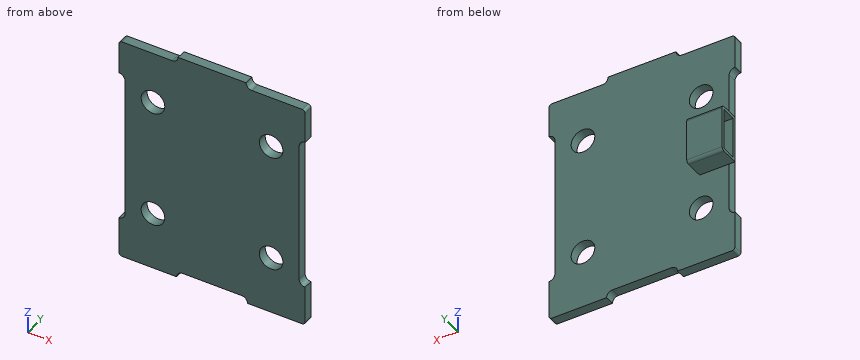
from build123d import *

# Parameters (mm, degrees)
SKETCH1_R           = 2
BOSS_EXTRUDE1_DEPTH = 1.6
SKETCH2_W           = 6
SKETCH2_H           = 8
BOSS_EXTRUDE2_DEPTH = 3.5
FILLET1_R           = 1
FILLET2_R           = 0.5
SKETCH3_W           = 7
SKETCH3_H           = 2.5
CUT_EXTRUDE1_DEPTH  = 5


with BuildPart() as part:
    # Sketch1 → Boss-Extrude1 (new body)
    with BuildSketch(Plane(origin=(0, 0, 0), x_dir=(1, 0, 0), z_dir=(0, 1, 0))):
        Polygon((15.75, 13), (15.75, 19.75), (6, 19.75), (6, 18.75), (-6, 18.75), (-6, 19.75), (-15.75, 19.75), (-15.75, 13), (-14.75, 13), (-14.75, -13), (-15.75, -13), (-15.75, -18.75), (-5.75, -18.75), (-5.75, -19.75), (5.75, -19.75), (5.75, -18.75), (15.75, -18.75), (15.75, -13), (14.75, -13), (14.75, 13), align=None)
        with Locations(Location((10, -10, 0), (0, 0, 270))):
            Circle(SKETCH1_R, mode=Mode.SUBTRACT)
        with Locations(Location((10, 10, 0), (0, 0, 270))):
            Circle(SKETCH1_R, mode=Mode.SUBTRACT)
        with Locations(Location((-10, 10, 0), (0, 0, 270))):
            Circle(SKETCH1_R, mode=Mode.SUBTRACT)
        with Locations(Location((-10, -10, 0), (0, 0, 270))):
            Circle(SKETCH1_R, mode=Mode.SUBTRACT)
    extrude(amount=BOSS_EXTRUDE1_DEPTH)

    # Sketch2 → Boss-Extrude2 (add)
    with BuildSketch(Plane(origin=(0, 1.6, 0), x_dir=(1, 0, 0), z_dir=(0, 1, 0))):
        with Locations((-12.75, 0)):
            Rectangle(SKETCH2_W, SKETCH2_H)
    extrude(amount=BOSS_EXTRUDE2_DEPTH)

    # Fillet1
    fillet1_edges = [part.edges().sort_by_distance(p)[0] for p in [
        (14.75, 0.8, -13),
        (14.75, 0.8, 13),
        (-6, 0.8, -18.75),
        (6, 0.8, -18.75),
        (-14.75, 0.8, -13),
        (-14.75, 0.8, 13),
        (-5.75, 0.8, 18.75),
        (5.75, 0.8, 18.75),
    ]]
    fillet(fillet1_edges, radius=FILLET1_R - 0.0001)  # a hair under: the kernel refuses the full size

    # Fillet2
    fillet2_edges = [part.edges().sort_by_distance(p)[0] for p in [
        (-15.75, 0.8, 18.75),
        (-15.75, 0.8, -19.75),
        (15.75, 0.8, -19.75),
        (15.75, 0.8, 18.75),
        (-12.75, 5.1, -4),
        (-12.75, 5.1, 4),
    ]]
    fillet(fillet2_edges, radius=FILLET2_R)

    # Sketch3 → Cut-Extrude1 (cut)
    with BuildSketch(Plane.ZY.offset(15.75)):
        with Locations((0, 3.35)):
            Rectangle(SKETCH3_W, SKETCH3_H)
    extrude(amount=-CUT_EXTRUDE1_DEPTH, mode=Mode.SUBTRACT)


solid = part.part
CAD build for the part. Positions are in the model's coordinates, mm. Give positions to 0.01 mm unless a question says otherwise; leave off trailing zeros. Order: outer loops, then holes, each group sorted by start corner. A loop starts at its lowest first (then second) coordinate and runs counter-clockwise, first axis right, second up. Notation, with made-up numbers: (41.5, 28.5) - (89.5, 28.5) arc R26 ccw to (89.5, 49.5) - close; hole circle Ø11 at (-0.5, 59.5). An arc over 180 degrees is marked (long way). Write each question's results on one line, items separated by ' | '.
1. Saw through at A-A on z = 10. List the corners of the cut face in (x, y), and give its area (3 significant figures).
Calculated:
outline: (-14.75, 0) - (-12, 0) - (-12, 1.6) - (-14.75, 1.6) - close; (-8, 0) - (8, 0) - (8, 1.6) - (-8, 1.6) - close; (12, 0) - (14.75, 0) - (14.75, 1.6) - (12, 1.6) - close | area: 34.4 mm2
2. Saw through at C-C on y = 3.65. List the corners of the cut face in (x, z).
Calculated:
outline: (-15.75, -4) - (-9.75, -4) - (-9.75, 4) - (-15.75, 4) - (-15.75, 3.5) - (-10.75, 3.5) - (-10.75, -3.5) - (-15.75, -3.5) - close
3. Saw through at D-D on z = -3. List the corners of the cut face in (x, y), and give its area (3 significant figures).
Calculated:
outline: (-15.75, 1.6) - (-14.75, 1.6) - (-14.75, 0) - (14.75, 0) - (14.75, 1.6) - (-9.75, 1.6) - (-9.75, 5.1) - (-15.75, 5.1) - (-15.75, 4.6) - (-10.75, 4.6) - (-10.75, 2.1) - (-15.75, 2.1) - close | area: 55.7 mm2
4. Probe L1, parallel to X at y = 0.9, z = -10; L2, parallel to Z at x = -11.5, y = 3.65; L3, parallel to X at y = 1.3, z = 9. List the from-to ranges inside material, lowest first. Write a range as from..to.
Calculated:
L1: x = -14.75..-12, -8..8, 12..14.75 | L2: z = -4..-3.5, 3.5..4 | L3: x = -14.75..-11.73, -8.27..8.27, 11.73..14.75
5. Saw through at B-B on x = 10. List the corners of the cut face in (y, z).
Calculated:
outline: (0, -19.75) - (1.6, -19.75) - (1.6, -12) - (0, -12) - close; (0, -8) - (1.6, -8) - (1.6, 8) - (0, 8) - close; (0, 12) - (1.6, 12) - (1.6, 18.75) - (0, 18.75) - close
6. Pin check, flat tips, straight feed: pin 1 (1.5 mm diameter, centred on x = -14, y = 3.5, fed in from +Z); pin 2 (1.8 mm diameter, centred on x = 2, y = 0.5, fed in from -Z); pin 3 (1.8 mm diameter, centred on y = 1, z = 3, fed in from +X); pin 4 (2 mm diameter, centred on x = 0, z = 13, fed in from -Y). Stop position of each tip, or through.
Calculated:
pin 1: stops at z = 4 | pin 2: stops at z = -18.75 | pin 3: stops at x = 14.75 | pin 4: stops at y = 0
